Can you work these out from the model? Positions are in its coordinate system, mm. Face numbers are marked on the shaded views. Coordinates: 2 decimals unless noted, no trailing zeros. Loops run counter-clockwise (first coordinate to the right, second up) from the corner with the lowest first, then second, coordinate; pieces in that order, holes last.
Autodesk Inventor part; units mm, degrees
ref_plane "YZ Plane" through (0, 0, 0) normal (1, 0, 0) x (0, 1, 0)
ref_plane "XZ Plane" through (0, 0, 0) normal (0, 1, 0) x (-1, 0, 0)
ref_plane "XY Plane" through (0, 0, 0) normal (0, 0, 1) x (1, 0, 0)
sketch "Sketch1" plane through (0, 0, 0) normal (0, 1, 0) x (-1, 0, 0)
  circle A0 centre (0, 0) radius 28
  dimension "d0" = 56
extrude "Extrusion1" add sketch "Sketch1" along normal mid plane 4
sketch "Sketch2" plane through (0, 2, 0) normal (0, 1, 0) x (1, 0, 0)
  circle A0 centre (0, 22.5) radius 2.05
  circle A1 centre (-15.9099, 15.9099) radius 2.05
  circle A2 centre (-22.5, 0) radius 2.05
  circle A3 centre (-15.9099, -15.9099) radius 2.05
  circle A4 centre (0, -22.5) radius 2.05
  circle A5 centre (15.9099, -15.9099) radius 2.05
  circle A6 centre (22.5, 0) radius 2.05
  circle A7 centre (15.9099, 15.9099) radius 2.05
  point P0 (0, 0)
  dimension "d3" = 4.1
  dimension "d4" = 22.5
  dimension "d7" = 360
extrude "Extrusion2" cut sketch "Sketch2" against normal through all
sketch "Sketch3" plane through (0, 2, 0) normal (0, 1, 0) x (1, 0, 0)
  circle A0 centre (0, 0) radius 16.1
  dimension "d11" = 32.2
extrude "Extrusion3" cut sketch "Sketch3" against normal through all
properties part number "BearingSpacerPlate"
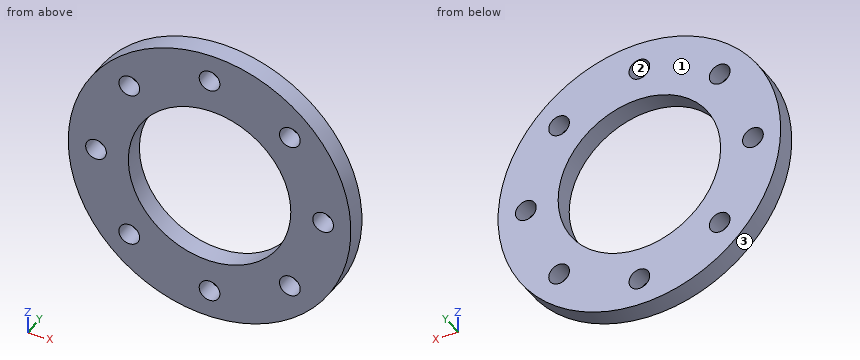
(1) I want a section at A-A on z = 0. Write out the boundary of the cut face in (x, y), then the cut area to 3 significant figures.
Check values:
outline: (-28, -2) - (-24.55, -2) - (-24.55, 2) - (-28, 2) - close; (-20.45, -2) - (-16.1, -2) - (-16.1, 2) - (-20.45, 2) - close; (16.1, -2) - (20.45, -2) - (20.45, 2) - (16.1, 2) - close; (24.55, -2) - (28, -2) - (28, 2) - (24.55, 2) - close
area: 62.4 mm2
(2) If I drill on probe 1 along Z at (x, y) = (0, 0.75); probe 2 along Z at (x, y) = (16.5, -0.2); probe 3 along Z at (x, y) = (4.5, 0.9), over which ranges is the centre line in solid material (lowest first)?
Check values:
probe 1: z = -28 to -24.55, -20.45 to -16.1, 16.1 to 20.45, 24.55 to 28
probe 2: z = -22.62 to -17.87, -13.95 to 13.95, 17.87 to 22.62
probe 3: z = -27.64 to -15.46, 15.46 to 27.64
(3) I want a section at C-C on x = 22.5. Write out the boundary of the cut face in (y, z), then the cut area to 3 significant figures.
Check values:
outline: (-2, -16.67) - (2, -16.67) - (2, -2.05) - (-2, -2.05) - close; (-2, 2.05) - (2, 2.05) - (2, 16.67) - (-2, 16.67) - close
area: 117 mm2
(4) I want a section at D-D on z = 21.5. Write out the boundary of the cut face in (x, y), then the cut area to 3 significant figures.
Check values:
outline: (-17.94, -2) - (-1.79, -2) - (-1.79, 2) - (-17.94, 2) - close; (1.79, -2) - (17.94, -2) - (17.94, 2) - (1.79, 2) - close
area: 129 mm2
(5) I want a section at B-B on x = 0. Write out the boundary of the cut face in (y, z), then the cut area to 3 significant figures.
Check values:
outline: (-2, -28) - (2, -28) - (2, -24.55) - (-2, -24.55) - close; (-2, -20.45) - (2, -20.45) - (2, -16.1) - (-2, -16.1) - close; (-2, 16.1) - (2, 16.1) - (2, 20.45) - (-2, 20.45) - close; (-2, 24.55) - (2, 24.55) - (2, 28) - (-2, 28) - close
area: 62.4 mm2
(6) If we mould it in two halves opening along X, with no side actions, what happens to the marked faces 1, 2 and 3? For each: released by +X, released by -X, zero draft, split by the parting line, or undercut.
Check values:
face 1: zero draft
face 2: undercut
face 3: split by the parting line
(7) I'm going to push flat-ended pins straight in: pin 1 (3.5 mm diameter, centred on x = 0, z = 22.5, fed in from +Y); pin 2 (2 mm diameter, centred on x = -6, y = -1.5, fed in from +Z); pin 3 (1 mm diameter, centred on y = 1.5, z = -18, fed in from -X). Where does each tip first touch, or does it pass through?
Check values:
pin 1: passes through
pin 2: stops at z = 27.55
pin 3: stops at x = -21.86
